Could you check a few things on this drawing? It's one solid part, dimensions in mm from its lowest x, y, z. A direction names the side the tool comes from. Give positions to 0.01 mm unless a question says otherwise; leave off trailing zeros. Loops run counter-clockwise (first coordinate to the right, second up) from the corner with the lowest first, then second, coordinate; pieces in that order, holes last. Notation, with made-up numbers: (-8.75, -5) - (15.25, -5) arc R21 cw to (15.25, 7) - close; hole circle Ø1 at (-6, 42.5). An arc over 180 degrees is marked (long way). Use a Markdown table: item, result.
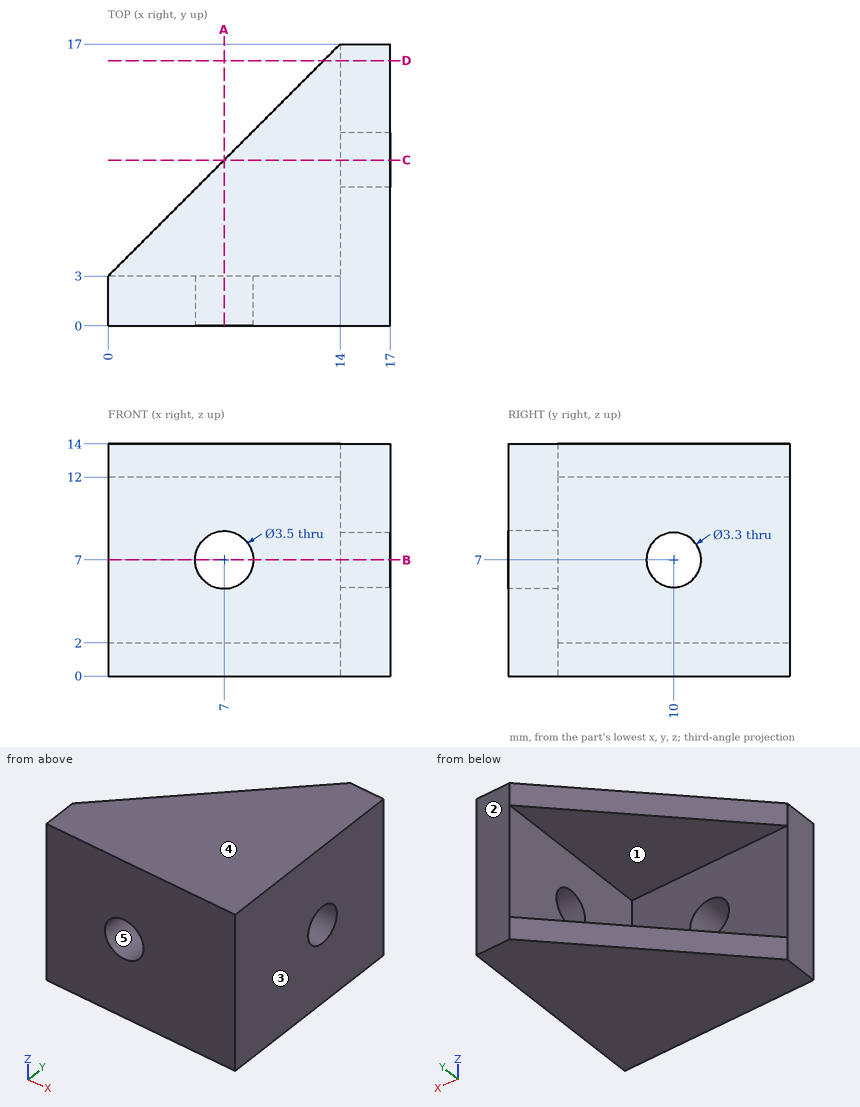
(1) Will these pins go through, and if not, where does the flat tip stop? pin 1 (3 mm diameter, centred on x = 9.5, z = 6, fed in from +Y); pin 2 (5 mm diameter, centred on y = 7, z = 5, fed in from -X).
A:
| item | result |
|---|---|
| pin 1 | y = 3 |
| pin 2 | x = 14 |
(2) Suppose I cut it at D-D on y = 16. Write out the boundary of the cut face in (x, z), plus the area to 3 significant figures.
A:
| item | result |
|---|---|
| outline | (13, 0) - (17, 0) - (17, 14) - (13, 14) - (13, 12) - (14, 12) - (14, 2) - (13, 2) - close |
| area | 46.0 mm2 |
(3) Suppose I cut it at C-C on y = 10. Write out the boundary of the cut face in (x, z).
A:
| item | result |
|---|---|
| outline | (7, 0) - (17, 0) - (17, 5.35) - (14, 5.35) - (14, 2) - (7, 2) - close; (7, 12) - (14, 12) - (14, 8.65) - (17, 8.65) - (17, 14) - (7, 14) - close |
(4) On a 3-axis mill with a long thin cutter (end or side, diameter ignored), from which of +Z, -Z, +X, -X, +Y, -Y can I reach the whole of each face in a straight line? I mean the marked faces 1 and 2. Say none if no direction works.
A:
| item | result |
|---|---|
| face 1 | -X, +Y |
| face 2 | +Z, -Z, +X, -X, +Y |
(5) Suppose I cut it at A-A on x = 7. Write out the boundary of the cut face in (y, z).
A:
| item | result |
|---|---|
| outline | (0, 0) - (10, 0) - (10, 2) - (3, 2) - (3, 5.25) - (0, 5.25) - close; (0, 8.75) - (3, 8.75) - (3, 12) - (10, 12) - (10, 14) - (0, 14) - close |
(6) Suppose I cut it at B-B on z = 7. Write out the boundary of the cut face in (x, y).
A:
| item | result |
|---|---|
| outline | (0, 0) - (5.25, 0) - (5.25, 3) - (0, 3) - close; (8.75, 0) - (17, 0) - (17, 8.35) - (14, 8.35) - (14, 3) - (8.75, 3) - close; (14, 11.65) - (17, 11.65) - (17, 17) - (14, 17) - close |
(7) We'd pull the mould along X, two halves only. Please class the marked faces 3, 4 and 5: pulls with the +X half, pulls with the -X half, needs draft (parallel to the pull), parting line crosses it, or undercut.
A:
| item | result |
|---|---|
| face 3 | pulls with the +X half |
| face 4 | needs draft |
| face 5 | undercut |
(8) If I drill on line 1 (Z direction, x = 7, y = 1.75); line 2 (Z direction, x = 13.75, y = 7.25); line 3 (Y direction, x = 16.15, z = 7), over which ranges is the centre line in solid material (lowest first)?
A:
| item | result |
|---|---|
| line 1 | 0 to 5.25, 8.75 to 14 |
| line 2 | 0 to 2, 12 to 14 |
| line 3 | 0 to 8.35, 11.65 to 17 |
